Design review of the part built by this model. Coordinates are the model's own, in mm. A direction names the side the tool comes from. Coordinates: 2 decimals unless noted, no trailing zeros. Loops run counter-clockwise (first coordinate to the right, second up) from the corner with the lowest first, then second, coordinate; pieces in that order, holes last. Notation, with made-up numbers: M 39.25,-9.5 L 66.25,-9.5 A22 cw 66.25,19.5 Z; hole C 60.5,1 d9. An arc over 180 degrees is marked long. One line per item, written item: value.
```python
from build123d import *

# Parameters (mm, degrees)
EXTRUDE_1_DEPTH = 2
SKETCH_2_R      = 0.75
EXTRUDE_2_DEPTH = 5
SKETCH_4_R      = 1
EXTRUDE_3_DEPTH = 5.5


with BuildPart() as part:
    # Эскиз1 → Бобышка-Вытянуть1 (new body)
    with BuildSketch(Plane.XY):
        with BuildLine():
            Line((-1.3027145, -2.134628779), (-3.80950787, -0.604790849))
            ThreePointArc((-3.80950787, -0.604790849), (-8.89711015, 0.858483074), (-14.018822021, -0.480522171))
            Line((-14.018822021, -0.480522171), (-16.936533206, -2.16506351))
            ThreePointArc((-16.936533206, -2.16506351), (-20.351596716, -1.25), (-19.436533206, 2.16506351))
            Line((-19.436533206, 2.16506351), (-16.593266604, 3.806624248))
            ThreePointArc((-16.593266604, 3.806624248), (-12.933012566, 7.466878286), (-11.593266604, 12.466878286))
            Line((-11.593266604, 12.466878286), (-11.593266604, 15.749999763))
            ThreePointArc((-11.593266604, 15.749999763), (-9.093266603, 18.249999764), (-6.593266603, 15.749999763))
            Line((-6.593266603, 15.749999763), (-6.593266603, 12.466878286))
            ThreePointArc((-6.593266603, 12.466878286), (-5.253520641, 7.466878286), (-1.593266603, 3.806624248))
            Line((-1.593266603, 3.806624248), (1.1972855, 2.19549824))
            ThreePointArc((1.1972855, 2.19549824), (2.165705155, -1.250370454), (-1.3027145, -2.134628779))
        make_face()
    extrude(amount=EXTRUDE_1_DEPTH)

    # Эскиз2 → Бобышка-Вытянуть2 (add)
    with BuildSketch(Plane(origin=(0, 0, 0), x_dir=(-1, 0, 0), z_dir=(0, 0, -1))):
        with Locations(Location((0, 0, 0), (0, 0, 180))):
            Circle(SKETCH_2_R)
        with Locations(Location((9.093266603, 15.749999763, 0), (0, 0, 180))):
            Circle(SKETCH_2_R)
        with Locations(Location((18.186533206, 0, 0), (0, 0, 180))):
            Circle(SKETCH_2_R)
    extrude(amount=EXTRUDE_2_DEPTH)

    # Эскиз4 → Бобышка-Вытянуть3 (add)
    with BuildSketch(Plane.XY.offset(2)):
        with Locations((-9.093266603, 5.249999921)):
            Circle(SKETCH_4_R)
    extrude(amount=EXTRUDE_3_DEPTH)


solid = part.part
```
(1) Tool access review of faces 1 (the flat face through (-15.457, -1.311, 0.986)), 2 (the cylindrical face through (-8.632, 4.363, 4.712)), 3 (the cylindrical face through (-17.471, -0.225, -2.465)): name each direction out of +Z, -Z, +X, -X, +Y, -Y from which nothing blocks a thin tool from reaching the whole face with its end or side.
Reply:
face 1: +Z, -Z, -Y
face 2: +Z
face 3: -Z
(2) Mouldability with a two-part tool opening along X and no side actions: class faces 4 (the flat face through (-0.2, 3, 1)), 5 (the flat face through (-2.54, -1.38, 0.99)), 6 (the flat face through (-18, 0, -5)), 7 (the cylindrical face through (-8.822, 0.857, 0.986)) as released by +X, released by -X, zero draft, split by the parting line, or undercut.
Reply:
face 4: released by +X
face 5: undercut
face 6: zero draft
face 7: undercut
(3) We need section C-C on z = 0.5. State the section outline as (x, y) points.
Reply:
outline: M -19.44,2.17 A2.5 ccw -16.94,-2.17 L -14.02,-0.48 A10 cw -3.81,-0.6 L -1.3,-2.13 A2.5 ccw long 1.2,2.2 L -1.59,3.81 A10 cw -6.59,12.47 L -6.59,15.75 A2.5 ccw -11.59,15.75 L -11.59,12.47 A10 cw -16.59,3.81 Z
(4) To check wall thickness, follow line 1 along Z through (x, y) = (-5.75, 5); line 2 along X through (y, z) = (14.5, 1.5); line 3 along Y through (x, z) = (-9.5, -0.75). State the ranges of each line that lie inside material, in increasing order. Write a range as [from, to].
Reply:
line 1: z = [0, 2]
line 2: x = [-11.59, -6.59]
line 3: y = [15.12, 16.38]
(5) Insertion check: pin 1 (1 mm diameter, centred on x = -12.5, y = 7, fed in from +Z); pin 2 (2 mm diameter, centred on y = 14, z = 1, fed in from +X); pin 3 (8 mm diameter, centred on x = -6, y = 1.5, fed in from -Z). Each pin has a flat end and moves straight along its axis. Give the tip position at first contact, or say it passes through.
Reply:
pin 1: stops at z = 2
pin 2: stops at x = -6.59
pin 3: stops at z = 0
(6) We need section D-D on y = 5.25. State the section outline as (x, z) points, then the cut area to 3 significant figures.
Reply:
outline: M -14.67,0 L -3.52,0 L -3.52,2 L -8.09,2 L -8.09,7.5 L -10.09,7.5 L -10.09,2 L -14.67,2 Z
area: 33.3 mm2
(7) We need section B-B on x = -9.5. State the section outline as (y, z) points.
Reply:
outline: M 0.85,0 L 15.12,0 L 15.12,-5 L 16.38,-5 L 16.38,0 L 18.22,0 L 18.22,2 L 6.16,2 L 6.16,7.5 L 4.34,7.5 L 4.34,2 L 0.85,2 Z
(8) We need section A-A on z = -1.75. State the section outline as (x, y) points.
Reply:
outline: C -18.19,0 d1.5; C -9.09,15.75 d1.5; C 0,0 d1.5
